Read the model definition and answer for the solid it produces. Units are mm, in the model's axes. A direction names the side the tool comes from. Give positions to 0.01 mm unless a question says otherwise; leave off trailing zeros. Write each question's results on one line, items separated by ' | '. Start each with the question number.
Q1. Given pin 1 (2 mm diameter, centred on x = -28, y = 31.5, fed in from +Z); pin 2 (8 mm diameter, centred on x = -20, y = 42.5, fed in from -Z); pin 3 (4 mm diameter, centred on x = 40, z = -28, fed in from +Y); pin 4 (4 mm diameter, centred on x = 44, z = 37, fed in from -Y), each flat-ended and moving along its own axis, determine where each tip first touches the part or whether it passes through.
Q2. Find the intervals of material crossed by line 1 (Z direction, x = 20, y = 35); line 2 (X direction, y = 53, z = -24.5); line 3 (Z direction, x = 0, y = 24), in increasing order. Write a range as from..to.
Q3. Determine the mould class of faces 3 (the flat face through (-9, 0, 52)), 4 (the flat face through (0, 8.925, -52)) for opening direction Z: +Z half, -Z half, draft (parallel to the pull), parting line (faces both ways), or undercut.
Q4. For faces 1 (the cylindrical face through (0.1, 18.9, -50.8)), 2 (the cylindrical face through (-17.659, 10.158, -48.297)), determine the directions among +Z, -Z, +X, -X, +Y, -Y from which every point of the face is accessible in a straight line to the end or side of a thin tool.
```python
from build123d import *

# Parameters (mm, degrees)
SKETCH_2_R               = 1.651
CUT_EXTRUDE_2_DEPTH      = 91.751697814
SKETCH_3_R               = 3.175
CUT_EXTRUDE_3_DEPTH      = 26
CUT_EXTRUDE_6_DEPTH      = 171.936937112
PATTERN_CIRCULAR_1_COUNT = 3


with BuildPart() as part:
    # 草图1 → 旋转1 (revolve)
    with BuildSketch(Plane.XY):
        with BuildLine():
            Line((-57.15, 0), (-48.201934037, 0))
            add(Edge.make_bspline(
                [(-48.201934037, 0), (-47.996267093, 1.778662864), (-47.522687895, 5.659356316), (-46.359317113, 13.861065304), (-44.38586856, 24.435820868), (-40.985955974, 36.381836571), (-36.337578012, 46.932872089), (-31.338663057, 54.099865092), (-26.597509905, 58.73057135), (-22.613977153, 61.657830569), (-18.108849913, 64.039104922), (-13.81197765, 65.548303683), (-9.980690551, 66.436316246), (-6.897059853, 66.930115728), (-4.135495293, 67.186856186), (-1.818265262, 67.292050819), (-0.601290545, 67.31), (0, 67.31)],
                knots=[0.009869614, 0.009869614, 0.009869614, 0.009869614, 0.0625, 0.125, 0.25, 0.375, 0.5, 0.625, 0.6875, 0.75, 0.8125, 0.875, 0.90625, 0.9375, 0.96875, 0.984375, 1, 1, 1, 1], degree=3))
            Line((0, 67.31), (0, 76.2))
            add(Edge.make_bspline(
                [(-57.15, 0), (-53.272554224, 34.209036409), (-44.696037368, 76.2), (0, 76.2)],
                knots=[0, 0, 0, 0, 1, 1, 1, 1], degree=3))
        make_face()
    revolve(axis=Axis((0, 0, 0), (0, 1, 0)))

    # 草图2 → 切除-拉伸2 (cut, through all)
    with BuildSketch(Plane(origin=(0, 34.925, 0), x_dir=(-1, 0, 0), z_dir=(0, -1, 0))):
        with Locations(Location((0, 53.975, 0), (0, 0, 270))):
            Circle(SKETCH_2_R)
    extrude(amount=CUT_EXTRUDE_2_DEPTH, mode=Mode.SUBTRACT)

    # 草图3 → 切除-拉伸3 (cut)
    with BuildSketch(Plane(origin=(0, 34.925, 0), x_dir=(-1, 0, 0), z_dir=(0, -1, 0))):
        with Locations((0, 53.975)):
            Circle(SKETCH_3_R)
    extrude(amount=CUT_EXTRUDE_3_DEPTH, mode=Mode.SUBTRACT)

    # 草图4 → 切除-拉伸6 (cut, through all)
    with BuildSketch(Plane(origin=(-78.631059864, 0, -13.394313695), x_dir=(0.16792488488501636, 0, -0.9857997935870925), z_dir=(0.9857997935870924, 0, 0.16792488488501633))):
        with BuildLine():
            Line((10.16, 0), (-10.16, 0))
            ThreePointArc((-10.16, 0), (0, 10.16), (10.16, 0))
        make_face()
    cut_extrude_6 = extrude(amount=CUT_EXTRUDE_6_DEPTH, mode=Mode.SUBTRACT)

    # 阵列(圆周)1: 切除-拉伸6 ×3 about axis
    pattern_circular_1_axis = Axis((0, 0, 0), (0, 1, 0))
    for i in range(1, PATTERN_CIRCULAR_1_COUNT):
        add(cut_extrude_6.rotate(pattern_circular_1_axis, i * 360 / PATTERN_CIRCULAR_1_COUNT), mode=Mode.SUBTRACT)


solid = part.part
```
Check sheet entries:
1) pin 1: stops at z = 44 | pin 2: stops at z = -45.85 | pin 3: stops at y = 44.98 | pin 4: stops at y = 0
2) line 1: z = -46.4..-36, 36..46.4 | line 2: x = -34.95..-20.44, 20.44..34.95 | line 3: z = -50.8..-44.29, 44.29..53.4
3) face 3: draft | face 4: undercut
4) face 1: +Y | face 2: -Y
